from build123d import *

# Parameters (mm, degrees)
F0_R     = 63.5
F1_DEPTH = 15.24
F2_SIZE2 = 27.94
F2_SIZE  = 7.4865004365
F3_R     = 22.86
F4_DEPTH = 25.4
F5_R     = 5.08


with BuildPart() as f1:
    # F0 (on Top) → F1 (new body)
    with BuildSketch(Plane.XY):
        Circle(F0_R)
    extrude(amount=F1_DEPTH)

    # F2
    f2_edges = [f1.edges().sort_by_distance(p)[0] for p in [
        (-63.5, 0, 15.24),
        (63.5, 0, 7.62),
        (-63.5, 0, 0),
    ]]
    f2_side = f1.faces().sort_by_distance((-63.5, 0, 7.62))[0]
    chamfer(f2_edges, length=F2_SIZE, length2=F2_SIZE2, reference=f2_side)

    # F3 (on face) → F4 (cut)
    with BuildSketch(Plane.XY.offset(15.24)):
        Circle(F3_R)
    extrude(amount=-F4_DEPTH, mode=Mode.SUBTRACT)

    # F5
    f5_edges = [f1.edges().sort_by_distance(p)[0] for p in [
        (-22.86, 0, 15.24),
        (-22.86, 0, 0),
    ]]
    fillet(f5_edges, radius=F5_R)


solid = f1.part
Check sheet for the modelled part. Datum: model origin and axes. Units: mm. Coordinates: 2 decimals unless noted, no trailing zeros. Loops run counter-clockwise (first coordinate to the right, second up) from the corner with the lowest first, then second, coordinate; pieces in that order, holes last. Notation, with made-up numbers: (-23.75, 56.5) -> (19.25, 56.5) arc R11 ccw to (19.25, 60.5) -> close; hole circle Ø11 at (85, 7.5). An arc over 180 degrees is marked (long way). Answer in a Markdown table with one row per item.
1. Go/stop test with flat-tipped pins: pin 1 (12 mm diameter, centred on x = 14.5, y = 50.5, fed in from +Z); pin 2 (6 mm diameter, centred on y = -1, z = 5, fed in from -X). Record where each tip stops, or that it passes through.
Check values:
| item | result |
|---|---|
| pin 1 | stops at z = 12.3 |
| pin 2 | stops at x = -63.5 |
2. Release check for a two-part mould opening along Y. For faces 1 (the face through (16, -24, 0)), 2 (the face through (19.846, 31.128, 0.364)), 3 (the face through (21.804, 6.867, 7.656)) record: released by +Y, released by -Y, zero draft, split by the parting line, or undercut.
Check values:
| item | result |
|---|---|
| face 1 | zero draft |
| face 2 | split by the parting line |
| face 3 | undercut |
3. Sectioned sample at C-C, the plane z = 3. Record the boundary of the cut face in (x, y).
Check values:
| item | result |
|---|---|
| outline | circle Ø93.51 at (0, 0); hole circle Ø46.61 at (0, 0) |
4. Sectioned sample at A-A, the plane x = 0. Record the boundary of the cut face in (y, z), then the cut area to 3 significant figures.
Check values:
| item | result |
|---|---|
| outline | (-63.5, 7.49) -> (-35.56, 0) -> (-27.94, 0) arc R5.08 ccw to (-22.86, 5.08) -> (-22.86, 10.16) arc R5.08 ccw to (-27.94, 15.24) -> (-35.56, 15.24) -> (-63.5, 7.75) -> close; (22.86, 5.08) arc R5.08 ccw to (27.94, 0) -> (35.56, 0) -> (63.5, 7.49) -> (63.5, 7.75) -> (35.56, 15.24) -> (27.94, 15.24) arc R5.08 ccw to (22.86, 10.16) -> close |
| area | 798 mm2 |
5. Sectioned sample at D-D, the plane z = 12. Record the boundary of the cut face in (x, y), then the cut area to 3 significant figures.
Check values:
| item | result |
|---|---|
| outline | circle Ø95.3 at (0, 0); hole circle Ø46.41 at (0, 0) |
| area | 5,440 mm2 |
6. Material ranges on line 1 along Z through (x, y) = (38, 12); line 2 along Z through (x, y) = (39, -6.5), recorded low to high. Write a range as [from, to].
Check values:
| item | result |
|---|---|
| line 1 | z = [1.15, 14.09] |
| line 2 | z = [1.07, 14.17] |
